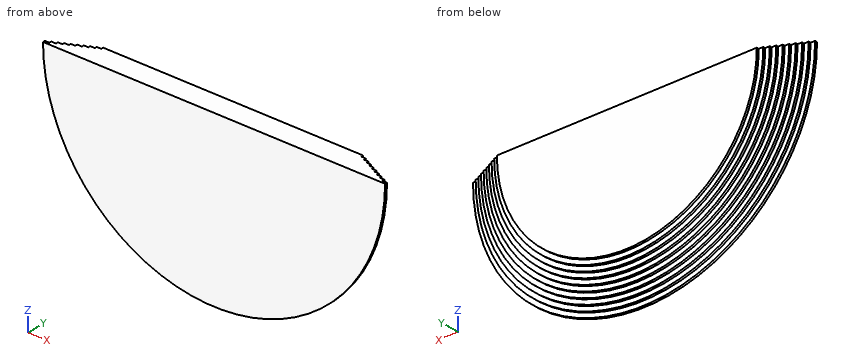
from build123d import *

# Parameters (mm, degrees)
EXTRUDE_1_DEPTH  = 0.2
EXTRUDE_3_DEPTH  = 0.2
EXTRUDE_4_DEPTH  = 0.2
EXTRUDE_5_DEPTH  = 0.2
EXTRUDE_6_DEPTH  = 0.2
EXTRUDE_7_DEPTH  = 0.2
EXTRUDE_8_DEPTH  = 0.2
EXTRUDE_9_DEPTH  = 0.2
EXTRUDE_10_DEPTH = 0.2
EXTRUDE_11_DEPTH = 0.2


with BuildPart() as part:
    # 草图1 → 凸台-拉伸1 (new body)
    with BuildSketch(Plane(origin=(0, 0, 0), x_dir=(1, 0, 0), z_dir=(0, 1, 0))):
        with BuildLine():
            Line((-15, 0), (15, 0))
            ThreePointArc((15, 0), (0, 15), (-15, 0))
        make_face()
    extrude(amount=EXTRUDE_1_DEPTH)

    # 草图2 → 凸台-拉伸3 (add)
    with BuildSketch(Plane(origin=(0, 0.2, 0), x_dir=(1, 0, 0), z_dir=(0, 1, 0))):
        with BuildLine():
            Line((-14.6, 0), (14.6, 0))
            ThreePointArc((14.6, 0), (0, 14.6), (-14.6, 0))
        make_face()
    extrude(amount=EXTRUDE_3_DEPTH)

    # 草图3 → 凸台-拉伸4 (add)
    with BuildSketch(Plane(origin=(0, 0.4, 0), x_dir=(1, 0, 0), z_dir=(0, 1, 0))):
        with BuildLine():
            Line((-14.2, 0), (14.2, 0))
            ThreePointArc((14.2, 0), (0, 14.2), (-14.2, 0))
        make_face()
    extrude(amount=EXTRUDE_4_DEPTH)

    # 草图4 → 凸台-拉伸5 (add)
    with BuildSketch(Plane(origin=(0, 0.6, 0), x_dir=(1, 0, 0), z_dir=(0, 1, 0))):
        with BuildLine():
            Line((-13.8, 0), (13.8, 0))
            ThreePointArc((13.8, 0), (0, 13.8), (-13.8, 0))
        make_face()
    extrude(amount=EXTRUDE_5_DEPTH)

    # 草图5 → 凸台-拉伸6 (add)
    with BuildSketch(Plane(origin=(0, 0.8, 0), x_dir=(1, 0, 0), z_dir=(0, 1, 0))):
        with BuildLine():
            Line((-13.4, 0), (13.4, 0))
            ThreePointArc((13.4, 0), (0, 13.4), (-13.4, 0))
        make_face()
    extrude(amount=EXTRUDE_6_DEPTH)

    # 草图6 → 凸台-拉伸7 (add)
    with BuildSketch(Plane(origin=(0, 1, 0), x_dir=(1, 0, 0), z_dir=(0, 1, 0))):
        with BuildLine():
            Line((-13, 0), (13, 0))
            ThreePointArc((13, 0), (0, 13), (-13, 0))
        make_face()
    extrude(amount=EXTRUDE_7_DEPTH)

    # 草图7 → 凸台-拉伸8 (add)
    with BuildSketch(Plane(origin=(0, 1.2, 0), x_dir=(1, 0, 0), z_dir=(0, 1, 0))):
        with BuildLine():
            Line((-12.6, 0), (12.6, 0))
            ThreePointArc((12.6, 0), (0, 12.6), (-12.6, 0))
        make_face()
    extrude(amount=EXTRUDE_8_DEPTH)

    # 草图8 → 凸台-拉伸9 (add)
    with BuildSketch(Plane(origin=(0, 1.4, 0), x_dir=(1, 0, 0), z_dir=(0, 1, 0))):
        with BuildLine():
            Line((-12.2, 0), (12.2, 0))
            ThreePointArc((12.2, 0), (0, 12.2), (-12.2, 0))
        make_face()
    extrude(amount=EXTRUDE_9_DEPTH)

    # 草图9 → 凸台-拉伸10 (add)
    with BuildSketch(Plane(origin=(0, 1.6, 0), x_dir=(1, 0, 0), z_dir=(0, 1, 0))):
        with BuildLine():
            Line((-11.8, 0), (11.8, 0))
            ThreePointArc((11.8, 0), (0, 11.8), (-11.8, 0))
        make_face()
    extrude(amount=EXTRUDE_10_DEPTH)

    # 草图10 → 凸台-拉伸11 (add)
    with BuildSketch(Plane(origin=(0, 1.8, 0), x_dir=(1, 0, 0), z_dir=(0, 1, 0))):
        with BuildLine():
            Line((-11.4, 0), (11.4, 0))
            ThreePointArc((11.4, 0), (0, 11.4), (-11.4, 0))
        make_face()
    extrude(amount=EXTRUDE_11_DEPTH)


solid = part.part
For this review, take the finished solid that the model builds, in its own axes (mm). Give positions to 0.01 mm unless a question says otherwise; leave off trailing zeros. Loops run counter-clockwise (first coordinate to the right, second up) from the corner with the lowest first, then second, coordinate; pieces in that order, holes last. Notation, with made-up numbers: (35.5, 17.25) -> (92.5, 17.25) arc R16 cw to (92.5, 35.25) -> close; hole circle Ø1 at (33.5, 4). An arc over 180 degrees is marked (long way). One line per question, with ' | ' between items.
1) To check wall thickness, follow probe 1 along Y at (x, z) = (-8, -8.75); probe 2 along Z at (x, y) = (6.75, 0.1); probe 3 along Y at (x, z) = (6, -11). State the ranges of each line that lie inside material, in increasing order.
Resolved:
probe 1: y = 0 to 1.6 | probe 2: z = -13.4 to 0 | probe 3: y = 0 to 1.4
2) We need section A-A (x = 1.75). Write out the cut boundary in (y, z), plus the area to 3 significant figures.
Resolved:
outline: (0, -14.9) -> (0.2, -14.9) -> (0.2, -14.49) -> (0.4, -14.49) -> (0.4, -14.09) -> (0.6, -14.09) -> (0.6, -13.69) -> (0.8, -13.69) -> (0.8, -13.29) -> (1, -13.29) -> (1, -12.88) -> (1.2, -12.88) -> (1.2, -12.48) -> (1.4, -12.48) -> (1.4, -12.07) -> (1.6, -12.07) -> (1.6, -11.67) -> (1.8, -11.67) -> (1.8, -11.26) -> (2, -11.26) -> (2, 0) -> (0, 0) -> close | area: 26.2 mm2
3) Insertion check: pin 1 Ø3 at (x, z) = (9, -5) entering from -Y. The pin has a flat end and moves straight along its axis. Give the tip position at first contact, or say it passes through.
Resolved:
pin 1: stops at y = 0
